Job drawing, mm, ordinate dimensions from the low corner. One solid piece. A direction names the side the tool comes from. Give positions to 0.01 mm unless a question says otherwise; leave off trailing zeros. Order: outer loops, then holes, each group sorted by start corner. A loop starts at its lowest first (then second) coordinate and runs counter-clockwise, first axis right, second up. Notation, with made-up numbers: (23.5, 71.5) - (41.5, 71.5) arc R21 ccw to (41.5, 80.5) - close; hole circle Ø1 at (69.25, -37). An arc over 180 degrees is marked (long way). Write each question's results on one line, items separated by ' | '. Start each with the question number.
1) Cut at D-D on y = 21. List the corners of the cut face in (x, z).
2) Cut at B-B on y = 13.5. List the corners of the cut face in (x, z).
3) Two-plate mould, pull along Y, no slides. Class the marked faces 1, 2 and 3: +Y half, -Y half, draft (parallel to the pull), parting line (faces both ways), or undercut.
4) Cut at A-A on x = 17.25. List the corners of the cut face in (y, z).
5) Drill centre lines: line 1 along Y through (x, z) = (22, 19.5); line 2 along Y through (x, z) = (17.25, 22.6); line 3 along Z through (x, y) = (11.5, 2.5). Where is each one in solid material? Low to high. Write a range as from..to.
6) Tool access for the marked faces 4 and 5: list every direction of +Z, -Z, +X, -X, +Y, -Y with a clear straight run to the whole face (end or side of a thin tool).
7) Drop flat-ended pins along their axis: pin 1 Ø2 at (y, z) = (5.5, 6.5) entering from +X; pin 2 Ø8 at (x, y) = (16, 13) entering from -Z. Give the stop position or say it passes through.
8) Cut at C-C on z = 1.5. List the corners of the cut face in (x, y).
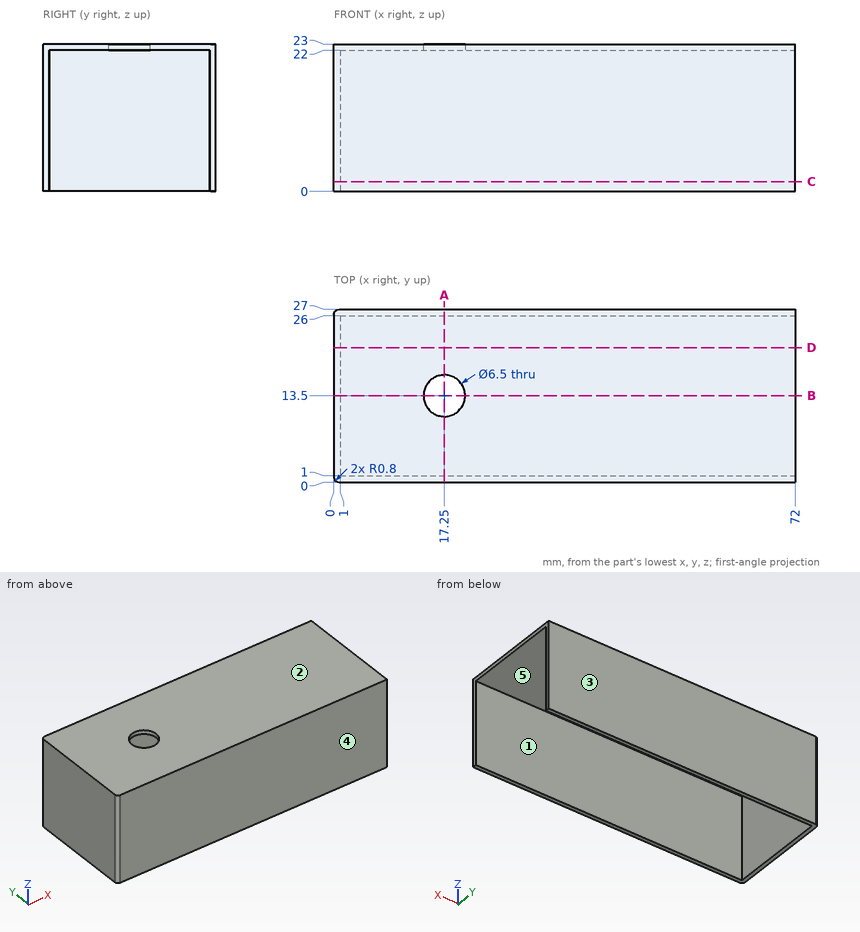
Results:
1) outline: (0, 0) - (1, 0) - (1, 22) - (72, 22) - (72, 23) - (0, 23) - close
2) outline: (0, 0) - (1, 0) - (1, 22) - (14, 22) - (14, 23) - (0, 23) - close; (20.5, 22) - (72, 22) - (72, 23) - (20.5, 23) - close
3) face 1: undercut | face 2: draft | face 3: +Y half
4) outline: (0, 0) - (1, 0) - (1, 22) - (10.25, 22) - (10.25, 23) - (0, 23) - close; (16.75, 22) - (26, 22) - (26, 0) - (27, 0) - (27, 23) - (16.75, 23) - close
5) line 1: 0..1, 26..27 | line 2: 0..10.25, 16.75..27 | line 3: 22..23
6) face 4: +Z, -Z, +X, -X, -Y | face 5: -Z, +X
7) pin 1: x = 1 | pin 2: z = 22
8) outline: (0, 0.8) arc R0.8 ccw to (0.8, 0) - (72, 0) - (72, 1) - (1, 1) - (1, 26) - (72, 26) - (72, 27) - (0.8, 27) arc R0.8 ccw to (0, 26.2) - close
